from build123d import *

# Parameters (mm, degrees)
SKETCH1_W           = 55
SKETCH1_H           = 64.43
BOSS_EXTRUDE1_DEPTH = 3
CUT_EXTRUDE1_DEPTH  = 4
SKETCH3_OUTSIDE_W   = 73.954
SKETCH3_OUTSIDE_H   = 83.384
CUT_EXTRUDE4_DEPTH  = 4
BOSS_EXTRUDE2_DEPTH = 3
BOSS_EXTRUDE3_DEPTH = 3
BOSS_EXTRUDE4_DEPTH = 4
BOSS_EXTRUDE5_DEPTH = 4
FILLET1_R           = 2
SKETCH9_R           = 1.75
CUT_EXTRUDE6_DEPTH  = 40.766745199
SKETCH10_R          = 3
CUT_EXTRUDE7_DEPTH  = 3
SKETCH11_R          = 1.75
CUT_EXTRUDE8_DEPTH  = 40.766745199


with BuildPart() as part:
    # Sketch1 → Boss-Extrude1 (new body)
    with BuildSketch(Plane(origin=(0, 0, 0), x_dir=(1, 0, 0), z_dir=(0, 1, 0))):
        Rectangle(SKETCH1_W, SKETCH1_H)
    extrude(amount=BOSS_EXTRUDE1_DEPTH)

    # Sketch2 → Cut-Extrude1 (cut)
    with BuildSketch(Plane(origin=(0, 3, 0), x_dir=(1, 0, 0), z_dir=(0, 1, 0))):
        Polygon((-27.5, -4.791277462), (-27.5, -14.373832386), (-17.5, -5), (-17.5, 5), (-27.5, 14.373832386), (-27.5, 4.791277462), align=None)
        Polygon((27.5, 4.791277462), (27.5, 14.373832386), (17.5, 5), (17.5, -5), (27.5, -14.373832386), (27.5, -4.791277462), align=None)
    extrude(amount=-CUT_EXTRUDE1_DEPTH, mode=Mode.SUBTRACT)

    # Sketch3 outside → Cut-Extrude4 (cut)
    with BuildSketch(Plane(origin=(0, 3, 0), x_dir=(1, 0, 0), z_dir=(0, 1, 0))):
        Rectangle(SKETCH3_OUTSIDE_W, SKETCH3_OUTSIDE_H)
        Polygon((-16, -5.649903378), (-16, 0), (-16, 5.649903378), (-25.681219861, 14.724916605), (-24.640371834, 16.957022404), (-9.782767538, 30.09765722), (-4.418267546, 24.032225889), (4.418267546, 24.032225889), (9.782767538, 30.09765722), (24.640371834, 16.957022404), (25.681219861, 14.724916605), (16, 5.649903378), (16, -5.649903378), (25.681219861, -14.724916605), (24.640371834, -16.957022404), (9.782767538, -30.09765722), (4.418267546, -24.032225889), (-4.418267546, -24.032225889), (-9.782767538, -30.09765722), (-24.640371834, -16.957022404), (-25.681219861, -14.724916605), align=None, mode=Mode.SUBTRACT)
    extrude(amount=-CUT_EXTRUDE4_DEPTH, mode=Mode.SUBTRACT)

    # Sketch4 → Boss-Extrude2 (add)
    with BuildSketch(Plane(origin=(0, 3, 0), x_dir=(1, 0, 0), z_dir=(0, 1, 0))):
        Polygon((-7.100517542, 27.064941555), (7.100517542, 27.064941555), (4.418267546, 24.032225889), (-4.418267546, 24.032225889), align=None)
        Polygon((-7.100517542, -27.064941555), (7.100517542, -27.064941555), (4.418267546, -24.032225889), (-4.418267546, -24.032225889), align=None)
    extrude(amount=-BOSS_EXTRUDE2_DEPTH)

    # Sketch5 → Boss-Extrude3 (add)
    with BuildSketch(Plane(origin=(0, 3, 0), x_dir=(1, 0, 0), z_dir=(0, 1, 0))):
        Polygon((-16, 5.649903378), (-18.188739123, 7.701590745), (-18.188739123, -7.701590745), (-16, -5.649903378), align=None)
        Polygon((16, 5.649903378), (18.188739123, 7.701590745), (18.188739123, -7.701590745), (16, -5.649903378), align=None)
    extrude(amount=-BOSS_EXTRUDE3_DEPTH)

    # Sketch6 → Boss-Extrude4 (add)
    with BuildSketch(Plane(origin=(0, 3, 0), x_dir=(1, 0, 0), z_dir=(0, 1, 0))):
        Polygon((-24.640371834, -16.957022404), (-25.681219861, -14.724916605), (-18.188739123, -7.701590745), (-18.188739123, 7.701590745), (-25.681219861, 14.724916605), (-24.640371834, 16.957022404), (-16, 8.373408054), (-16, -8.373408054), align=None)
        Polygon((16, -8.373408054), (24.640371834, -16.957022404), (25.681219861, -14.724916605), (18.188739123, -7.701590745), (18.188739123, 7.701590745), (25.681219861, 14.724916605), (24.640371834, 16.957022404), (16, 8.373408054), align=None)
    extrude(amount=BOSS_EXTRUDE4_DEPTH)

    # Sketch7 → Boss-Extrude5 (add)
    with BuildSketch(Plane(origin=(0, 3, 0), x_dir=(1, 0, 0), z_dir=(0, 1, 0))):
        Polygon((-1, 27.064941555), (-7.100517542, 27.064941555), (-9.782767538, 30.09765722), (-11.280892286, 28.772658262), (-7.100517542, 24.594941555), (-1, 24.594941555), (1, 24.594941555), (7.100517542, 24.594941555), (11.280892286, 28.772658262), (9.782767538, 30.09765722), (7.100517542, 27.064941555), (1, 27.064941555), align=None)
        Polygon((-1, -27.064941555), (-7.100517542, -27.064941555), (-9.782767538, -30.09765722), (-11.280892286, -28.772658262), (-7.100517542, -24.594941555), (-1, -24.594941555), (1, -24.594941555), (7.100517542, -24.594941555), (11.280892286, -28.772658262), (9.782767538, -30.09765722), (7.100517542, -27.064941555), (1, -27.064941555), align=None)
    extrude(amount=BOSS_EXTRUDE5_DEPTH)

    # Fillet1
    fillet1_edges = [part.edges().sort_by_distance(p)[0] for p in [
        (0, 0, -27.064941555),
        (0, 0, 27.064941555),
        (-21.934979492, 0, 11.213253675),
        (-21.934979492, 0, -11.213253675),
        (21.934979492, 0, -11.213253675),
        (21.934979492, 0, 11.213253675),
        (-18.188739123, 0, 0),
        (18.188739123, 0, 0),
        (-25.160795848, 0, 15.840969504),
        (-17.211569686, 0, 23.527339812),
        (-8.44164254, 0, 28.581299387),
        (8.44164254, 0, 28.581299387),
        (17.211569686, 0, 23.527339812),
        (25.160795848, 0, 15.840969504),
        (25.160795848, 0, -15.840969504),
        (17.211569686, 0, -23.527339812),
        (8.44164254, 0, -28.581299387),
        (-8.44164254, 0, -28.581299387),
        (-17.211569686, 0, -23.527339812),
        (-25.160795848, 0, -15.840969504),
    ]]
    fillet(fillet1_edges, radius=FILLET1_R)

    # Sketch9 → Cut-Extrude6 (cut, through all)
    with BuildSketch(Plane(origin=(0, 3, 0), x_dir=(1, 0, 0), z_dir=(0, 1, 0))):
        with Locations(Location((15.251219861, -15.244152763, 0), (0, 0, 270))):
            Circle(SKETCH9_R)
        with Locations(Location((15.251219861, 15.255847237, 0), (0, 0, 270))):
            Circle(SKETCH9_R)
        with Locations(Location((-15.248780139, 15.255847237, 0), (0, 0, 270))):
            Circle(SKETCH9_R)
        with Locations(Location((-15.248780139, -15.244152763, 0), (0, 0, 270))):
            Circle(SKETCH9_R)
    extrude(amount=-CUT_EXTRUDE6_DEPTH, mode=Mode.SUBTRACT)

    # Sketch10 → Cut-Extrude7 (cut)
    with BuildSketch(Plane.XZ):
        with Locations(Location((-15.248780139, -15.255847237, 0), (0, 0, 270))):
            Circle(SKETCH10_R)
        with Locations(Location((-15.248780139, 15.255847237, 0), (0, 0, 90))):
            Circle(SKETCH10_R)
        with Locations(Location((15.248780139, -15.255847237, 0), (0, 0, 90))):
            Circle(SKETCH10_R)
        with Locations(Location((15.248780139, 15.255847237, 0), (0, 0, 270))):
            Circle(SKETCH10_R)
    extrude(amount=-CUT_EXTRUDE7_DEPTH, mode=Mode.SUBTRACT)

    # Sketch11 → Cut-Extrude8 (cut, through all)
    with BuildSketch(Plane(origin=(0, 3, 0), x_dir=(1, 0, 0), z_dir=(0, 1, 0))):
        with Locations(Location((11.958739123, -5.07, 0), (0, 0, 270))):
            Circle(SKETCH11_R)
        with Locations(Location((11.958739123, 5.07, 0), (0, 0, 270))):
            Circle(SKETCH11_R)
        with Locations(Location((-11.958739123, -5.07, 0), (0, 0, 270))):
            Circle(SKETCH11_R)
        with Locations(Location((-11.958739123, 5.07, 0), (0, 0, 270))):
            Circle(SKETCH11_R)
    extrude(amount=-CUT_EXTRUDE8_DEPTH, mode=Mode.SUBTRACT)


solid = part.part
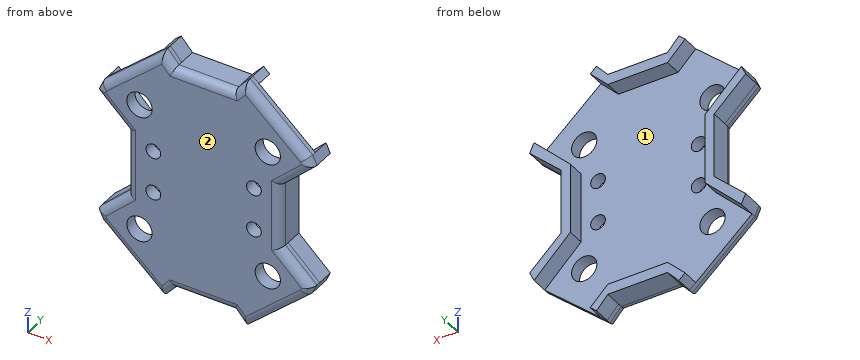
Geometry check sheet. Reference: the model listing, model coordinates, mm. Face numbers are marked on the shaded views. Round coordinates to 2 decimals unless told otherwise and drop trailing zeros. Order: outer loops, then holes, each group sorted by start corner. A loop starts at its lowest first (then second) coordinate and runs counter-clockwise, first axis right, second up. Notation, with made-up numbers: M -2.75,37.25 L 21.25,37.25 A12 cw 21.25,52.25 Z; hole C 9.5,80 d11. An arc over 180 degrees is marked long. Answer in a Markdown table with one row per item. Add a question column.
Item 1: Sectioned sample at B-B, the plane z = 5.07. Enter the section's corners in (x, y), plus the area to 3 significant figures.
Item 2: Sectioned sample at C-C, the plane x = 6. Enter the section's corners in (y, z).
Item 3: Sectioned sample at A-A, the plane y = 3.75. State how many separate pieces and enclosed holes the cut face has, plus the area to 3 significant figures.
Item 4: Draft check along X on the marked faces 1 and 2. Enter one of: released by +X, released by -X, zero draft, split by the parting line, or undercut.
Item 5: Depth check by flat-ended pin: pin 1 Ø2 at (x, y) = (-2.5, 5.5) entering from -Z; pin 2 Ø5.5 at (x, z) = (-11.96, 5.07) entering from +Y; pin 3 Ø2 at (x, z) = (-11.96, -5.07) entering from -Y; pin 4 Ø2 at (y, z) = (5.5, 1.5) entering from -X. Enter the tip coordinate at first touch or a pass-through.
Item 6: Material ranges on L1, parallel to Z at x = -4.5, y = 5.75; L2, parallel to X at y = 5.25, z = -2; L3, parallel to X at y = 0.5, z = 13.5, recorded low to high. Write a range as [from, to].
Filled in:
| question | item | result |
|---|---|---|
| 1 | outline | M -18.19,2 A2 ccw -16.19,0 L -13.71,0 L -13.71,3 L -16,3 L -16,7 L -18.19,7 Z; M -10.21,0 L 10.21,0 L 10.21,3 L -10.21,3 Z; M 13.71,0 L 16.19,0 A2 ccw 18.19,2 L 18.19,7 L 16,7 L 16,3 L 13.71,3 Z |
| 1 | area | 104 mm² |
| 2 | outline | M 0,-25.06 A2 ccw 2,-27.06 L 7,-27.06 L 7,-24.59 L 3,-24.59 L 3,24.59 L 7,24.59 L 7,27.06 L 2,27.06 A2 ccw 0,25.06 Z |
| 3 | separate pieces | 4 |
| 3 | enclosed holes | 0 |
| 3 | area | 275 mm² |
| 4 | face 1 | undercut |
| 4 | face 2 | zero draft |
| 5 | pin 1 | stops at z = -27.06 |
| 5 | pin 2 | stops at y = 3 |
| 5 | pin 3 | passes through |
| 5 | pin 4 | stops at x = -18.19 |
| 6 | L1 | z = [-27.06, -24.59], [24.59, 27.06] |
| 6 | L2 | x = [-18.19, -16], [16, 18.19] |
| 6 | L3 | x = [-23.38, -17.68], [-12.82, 12.82], [17.68, 23.38] |
